Input: part model. Units: mm. Frame: model coordinates. Face numbers are marked on the shaded views. A direction names the side the tool comes from. Coordinates: 2 decimals unless noted, no trailing zeros. Write each loop counter-clockwise with the first axis right and the second up, starting at its lowest first coordinate (ties: lowest second). Pieces come first, ordered by that corner, then holes. Notation, with made-up numbers: (79.5, -38.75) - (110.5, -38.75) arc R19 ccw to (110.5, -10.75) - close; hole circle Ø11 at (65.25, 69.5). An arc over 180 degrees is marked (long way). One line per question, with ' | ' between items. Start each with the question number.
1) First-contact query: P1, Ø17, axis at x = 0, y = -34.925, coming from the +Z side; P2, Ø5, axis at x = 20.51, y = 20.51, coming from the +Z side; P3, Ø4, axis at x = -2, z = -4, coming from the +Y side; P4, Ø2, axis at x = -14, y = -1.5, coming from the -Z side. Flat tips, straight axial feed; report the tip coordinate or a pass-through.
2) Section query C-C on y = 0. Return loops of the section in (x, z).
3) Line query: line 1 (X direction, y = -50.8, z = -5); line 2 (Y direction, x = 21.5, z = -4.25); line 3 (Y direction, x = -21, z = -3.75). Output: solid intervals per line, ascending.
4) Draft query along Y for the marked faces 4, 5, 6 and 7. Return one class per face: released by +Y, released by -Y, zero draft, split by the parting line, or undercut.
5) Section query B-B on x = 0. Return loops of the section in (y, z).
6) Reachability of the marked faces 1, 2 and 3 from +Z, -Z, +X, -X, +Y, -Y: full face, straight path, thin tool, end or side. Return the list, or none.
7) Section query A-A on y = -50.8. Give the number of separate pieces and of enclosed holes in the cut face, and give its area (3 significant figures).
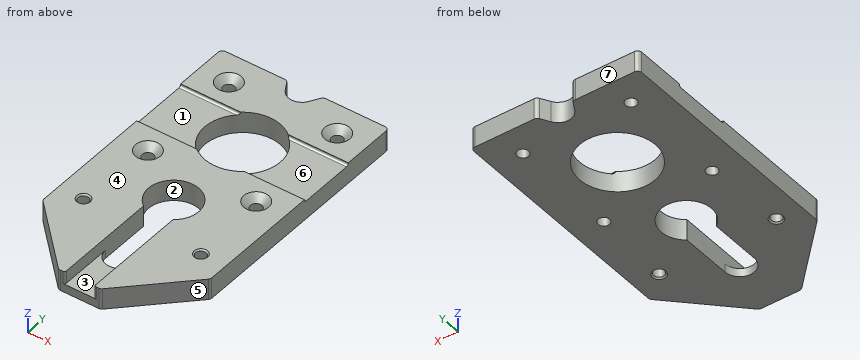
```python
from build123d import *

# Parameters (mm, degrees)
SKETCH1_R                                       = 14.2875
BOSS_EXTRUDE1_DEPTH                             = 7.9502
CUT_EXTRUDE1_DEPTH                              = 4.7752
CSK_FOR_M4_FLAT_HEAD_MACHINE_SCREW1_D           = 4.3
CSK_FOR_M4_FLAT_HEAD_MACHINE_SCREW1_CSINK_D     = 9.4
CSK_FOR_M4_FLAT_HEAD_MACHINE_SCREW1_CSINK_ANGLE = 90
CIRPATTERN1_COUNT                               = 4
F_10_32_TAPPED_HOLE1_AT_2_COUNT                 = 2
F_10_32_TAPPED_HOLE1_AT_2_PITCH                 = 44.45
CUT_EXTRUDE2_DEPTH                              = 89.801861918
FILLET1_R                                       = 1.5748
FILLET2_R                                       = 0.762
SKETCH12_W                                      = 73.210736231
SKETCH12_H                                      = 22.225
CUT_EXTRUDE3_DEPTH                              = 1.016
FILLET3_R                                       = 0.889


with BuildPart() as part:
    # Sketch1 → Boss-Extrude1 (new body)
    with BuildSketch(Plane.XY):
        Polygon((-31.75, 31.75), (31.75, 31.75), (31.75, -58.7248), (7.9248, -82.55), (-7.9248, -82.55), (-31.75, -58.7248), align=None)
        Circle(SKETCH1_R, mode=Mode.SUBTRACT)
        with BuildLine():
            Line((5.5626, -42.656953585), (5.5626, -61.9125))
            ThreePointArc((5.5626, -61.9125), (0, -67.4751), (-5.5626, -61.9125))
            Line((-5.5626, -61.9125), (-5.5626, -42.656953585))
            ThreePointArc((-5.5626, -42.656953585), (0, -25.4), (5.5626, -42.656953585))
        make_face(mode=Mode.SUBTRACT)
    extrude(amount=-BOSS_EXTRUDE1_DEPTH)

    # Sketch4 → Cut-Extrude1 (cut)
    with BuildSketch(Plane.XY):
        with BuildLine():
            Line((5.5626, -111.125), (5.5626, -34.925))
            ThreePointArc((5.5626, -34.925), (0, -29.3624), (-5.5626, -34.925))
            Line((-5.5626, -34.925), (-5.5626, -111.125))
            Line((-5.5626, -111.125), (5.5626, -111.125))
        make_face()
    extrude(amount=-CUT_EXTRUDE1_DEPTH, mode=Mode.SUBTRACT)

    # CSK for M4 Flat Head Machine Screw1 (through all)
    with Locations(Plane.XY):
        with Locations((20.506096654, 20.506096654)):
            csk_for_m4_flat_head_machine_screw1 = CounterSinkHole(CSK_FOR_M4_FLAT_HEAD_MACHINE_SCREW1_D / 2, CSK_FOR_M4_FLAT_HEAD_MACHINE_SCREW1_CSINK_D / 2, counter_sink_angle=CSK_FOR_M4_FLAT_HEAD_MACHINE_SCREW1_CSINK_ANGLE)

    # CirPattern1: CSK for M4 Flat Head Machine Screw1 ×4 about axis
    cirpattern1_axis = Axis((0, 0, 0), (0, 0, 1))
    for i in range(1, CIRPATTERN1_COUNT):
        add(csk_for_m4_flat_head_machine_screw1.rotate(cirpattern1_axis, i * 360 / CIRPATTERN1_COUNT), mode=Mode.SUBTRACT)

    # Sketch7 → #10-32 Tapped Hole1 (revolve, cut)
    with BuildSketch(Plane(origin=(22.225, -50.8, 0), x_dir=(0, -1, 0), z_dir=(1, 0, 0))):
        Polygon((0, 0), (0, 7.9502), (2.54, 7.9502), (2.0193, 7.4295), (2.0193, 0.5207), (2.54, 0), align=None)
    f_10_32_tapped_hole1 = revolve(axis=Axis((22.225, -50.8, 6.35), (0, 0, -1)), mode=Mode.SUBTRACT)

    # #10-32 Tapped Hole1 at 2: #10-32 Tapped Hole1 ×2
    with Locations(*[(-i * F_10_32_TAPPED_HOLE1_AT_2_PITCH, 0, 0) for i in range(1, F_10_32_TAPPED_HOLE1_AT_2_COUNT)]):
        add(f_10_32_tapped_hole1, mode=Mode.SUBTRACT)

    # Sketch8 → Cut-Extrude2 (cut, through all)
    with BuildSketch(Plane.XY):
        with BuildLine():
            Line((-4.465400187, 27.5971), (-13.062271505, 42.487317908))
            Line((-13.062271505, 42.487317908), (13.062271505, 42.487317908))
            Line((13.062271505, 42.487317908), (4.465400187, 27.5971))
            ThreePointArc((4.465400187, 27.5971), (0, 25.019), (-4.465400187, 27.5971))
        make_face()
    extrude(amount=-CUT_EXTRUDE2_DEPTH, mode=Mode.SUBTRACT)

    # Fillet1
    fillet1_edges = [part.edges().sort_by_distance(p)[0] for p in [
        (-31.75, 31.75, -3.9751),
        (31.75, 31.75, -3.9751),
        (31.75, -58.7248, -3.9751),
        (7.9248, -82.55, -3.9751),
        (-7.9248, -82.55, -3.9751),
        (-31.75, -58.7248, -3.9751),
        (-6.86307812, 31.75, -3.9751),
        (6.86307812, 31.75, -3.9751),
    ]]
    fillet(fillet1_edges, radius=FILLET1_R)

    # Fillet2
    fillet2_edges = [part.edges().sort_by_distance(p)[0] for p in [
        (-5.5626, -82.55, -2.3876),
        (5.5626, -82.55, -2.3876),
    ]]
    fillet(fillet2_edges, radius=FILLET2_R)

    # Sketch12 → Cut-Extrude3 (cut)
    with BuildSketch(Plane.XY):
        with Locations((0.072940044, 0)):
            Rectangle(SKETCH12_W, SKETCH12_H)
    extrude(amount=-CUT_EXTRUDE3_DEPTH, mode=Mode.SUBTRACT)

    # Fillet3
    fillet3_edges = [part.edges().sort_by_distance(p)[0] for p in [
        (20.365128061, -11.1125, -1.016),
        (-20.365128061, -11.1125, -1.016),
        (-20.365128061, 11.1125, -1.016),
        (20.365128061, 11.1125, -1.016),
    ]]
    fillet(fillet3_edges, radius=FILLET3_R)


solid = part.part
```
Answer key:
1) P1: through | P2: z = -2.19 | P3: y = 26.92 | P4: z = -7.95
2) outline: (-31.75, -7.95) - (-14.29, -7.95) - (-14.29, -1.02) - (-31.75, -1.02) - close; (14.29, -7.95) - (31.75, -7.95) - (31.75, -1.02) - (14.29, -1.02) - close
3) line 1: -31.75 to -24.24, -20.21 to -5.56, 5.56 to 20.21, 24.24 to 31.75 | line 2: -68.97 to -52.68, -48.92 to -22.41, -18.6 to 18.6, 22.41 to 31.75 | line 3: -69.47 to -52.41, -49.19 to -22.6, -18.41 to 18.41, 22.6 to 31.75
4) face 4: zero draft | face 5: released by -Y | face 6: undercut | face 7: released by +Y
5) outline: (-82.55, -7.95) - (-67.48, -7.95) - (-67.48, -4.78) - (-82.55, -4.78) - close; (-25.4, -7.95) - (-14.29, -7.95) - (-14.29, 0) - (-25.4, 0) - close; (14.29, -7.95) - (25.02, -7.95) - (25.02, 0) - (14.29, 0) - close
6) face 1: +Z, +X, -X | face 2: +Z, -Z | face 3: +Z, -Y
7) separate pieces: 4 | enclosed holes: 0 | area: 351 mm²
